Geometry check sheet. Reference: drawing and pictorial views, mm from the part's lowest x, y, z. Round coordinates to 2 decimals unless told otherwise and drop trailing zeros. Loops run counter-clockwise (first coordinate to the right, second up) from the corner with the lowest first, then second, coordinate; pieces in that order, holes last. Notation, with made-up numbers: (8, 39.25) - (51, 39.25) arc R36 ccw to (51, 76.25) - close; hole circle Ø3 at (64, 82). An arc over 180 degrees is marked (long way). Answer in a Markdown table with one row per item. Add a question column.
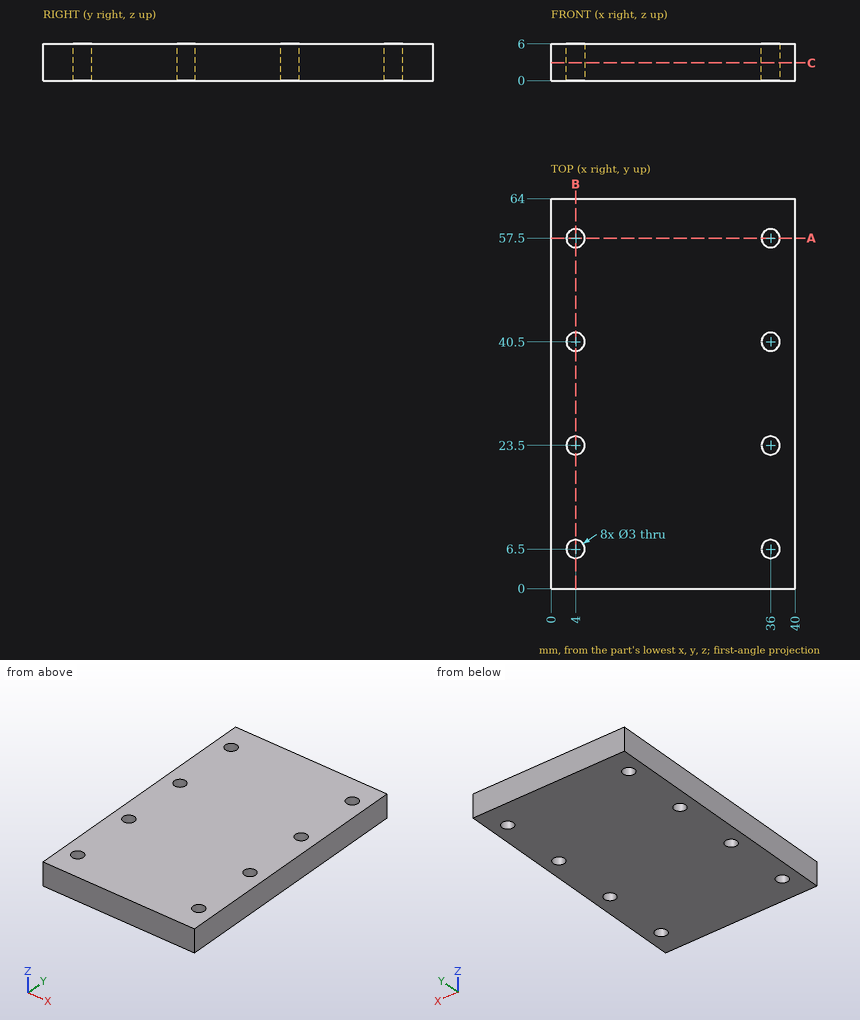
Q1. Cross-section at C-C, the plane z = 2.9. State how many separate pieces and enclosed holes the cut face has, plus the area to 3 significant figures.
Q2. Scan lines: line 1 (Y direction, x = 4, z = 4.2); line 2 (Y direction, x = 4.5, z = 5.1). Record each from-to range of solid material in increasing order. Write a range as from..to.
Q3. Cross-section at A-A, the plane y = 57.5. Enter the section's corners in (x, z).
Q4. Depth check by flat-ended pin: P1, Ø2.5, axis at x = 36, y = 40.5, coming from the -Z side. Enter the tip coordinate at first touch or a pass-through.
Q5. Cross-section at B-B, the plane x = 4. Enter the section's corners in (y, z), plus the area to 3 significant figures.
Check sheet entries:
| question | item | result |
|---|---|---|
| 1 | separate pieces | 1 |
| 1 | enclosed holes | 8 |
| 1 | area | 2,500 mm² |
| 2 | line 1 | 0..5, 8..22, 25..39, 42..56, 59..64 |
| 2 | line 2 | 0..5.09, 7.91..22.09, 24.91..39.09, 41.91..56.09, 58.91..64 |
| 3 | outline | (0, 0) - (2.5, 0) - (2.5, 6) - (0, 6) - close; (5.5, 0) - (34.5, 0) - (34.5, 6) - (5.5, 6) - close; (37.5, 0) - (40, 0) - (40, 6) - (37.5, 6) - close |
| 4 | P1 | through |
| 5 | outline | (0, 0) - (5, 0) - (5, 6) - (0, 6) - close; (8, 0) - (22, 0) - (22, 6) - (8, 6) - close; (25, 0) - (39, 0) - (39, 6) - (25, 6) - close; (42, 0) - (56, 0) - (56, 6) - (42, 6) - close; (59, 0) - (64, 0) - (64, 6) - (59, 6) - close |
| 5 | area | 312 mm² |
